Verification items for this drawing (mm, ordinates from the low corner). Coordinates: 2 decimals unless noted, no trailing zeros. Write each loop counter-clockwise with the first axis right and the second up, starting at its lowest first coordinate (ties: lowest second). Pieces come first, ordered by that corner, then holes.
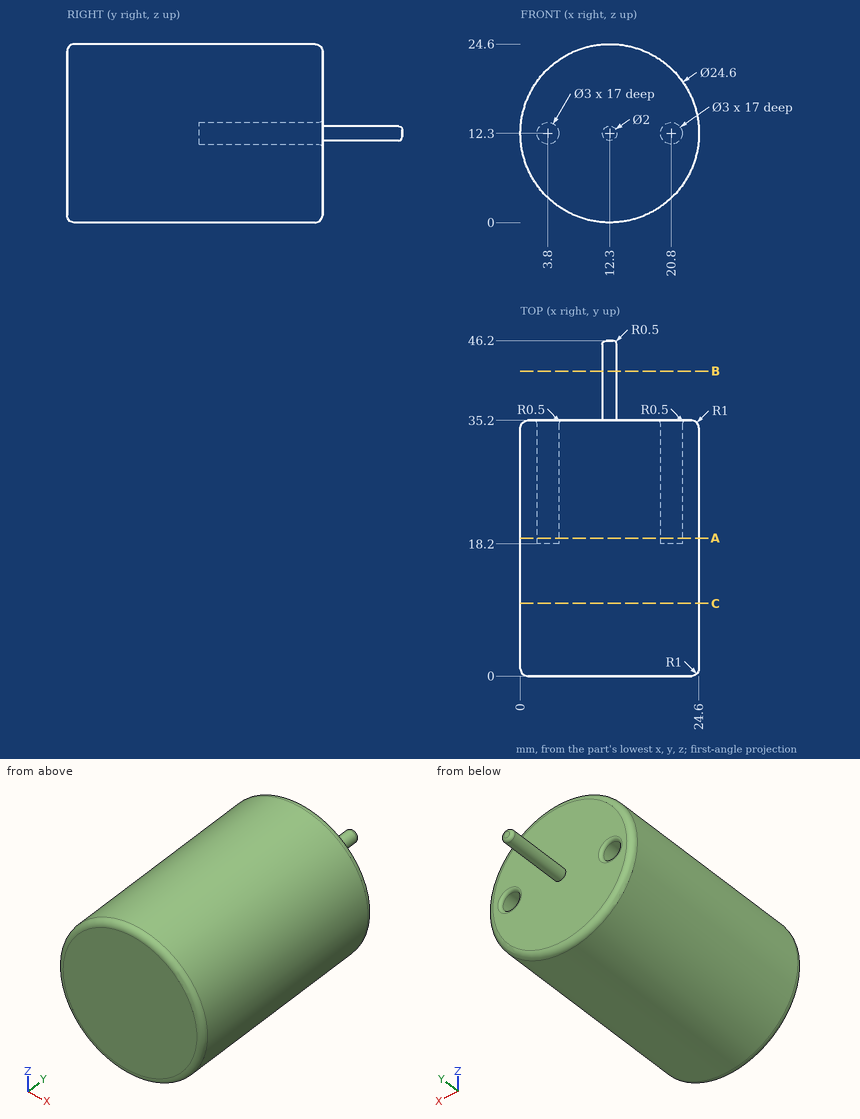
1. Thickness scan on line 1 along Y through (x, z) = (16.5, 19.25); line 2 along Z through (x, y) = (20.8, 28.75); line 3 along Z through (x, y) = (3.25, 22). Record the ranges inside material, lowest first.
Computed values:
line 1: y = 0 to 35.2
line 2: z = 3.41 to 10.8, 13.8 to 21.19
line 3: z = 3.97 to 10.9, 13.7 to 20.63
2. Sectioned sample at A-A, the plane y = 19. Record the boundary of the cut face in (x, z).
Computed values:
outline: circle Ø24.6 at (12.3, 12.3); hole circle Ø3 at (3.8, 12.3); hole circle Ø3 at (20.8, 12.3)
3. Sectioned sample at C-C, the plane y = 10. Record the boundary of the cut face in (x, z).
Computed values:
outline: circle Ø24.6 at (12.3, 12.3)
4. Gauge pin test, flat ends, axial feed: pin 1 Ø1.5 at (y, z) = (27.5, 14) entering from +X; pin 2 Ø2.5 at (x, z) = (3.8, 12.3) entering from +Y; pin 3 Ø2.5 at (x, z) = (20, 12.5) entering from +Y. Record the tip position at first contact, or that the pin passes through.
Computed values:
pin 1: stops at x = 24.56
pin 2: stops at y = 18.2
pin 3: stops at y = 35.2
5. Sectioned sample at B-B, the plane y = 42. Record the boundary of the cut face in (x, z), and give its area (3 significant figures).
Computed values:
outline: circle Ø2 at (12.3, 12.3)
area: 3.14 mm2
